Verification items for the finished model (mm, model axes). Coordinates: 2 decimals unless noted, no trailing zeros. Order: outer loops, then holes, each group sorted by start corner. A loop starts at its lowest first (then second) coordinate and runs counter-clockwise, first axis right, second up. Notation, with made-up numbers: (-23, 33) -> (9, 33) arc R28 ccw to (9, 54) -> close; hole circle Ø8 at (-31.75, 88.25). An arc over 180 degrees is marked (long way). Write each question's results on one line, items separated by ' | '. Start each with the question number.
(1) Go/stop test with a flat-tipped pin: pin 1 (6.5 mm diameter, centred on x = -41.5, z = 19.5, fed in from +Y). Record where the tip stops, or that it passes through.
(2) Cross-section at B-B on x = 0. Enter the section's corners in (y, z), and give its area (3 significant figures).
(3) Cross-section at C-C on z = 0. Enter the section's corners in (x, y), and give its area (3 significant figures).
(4) Cross-section at D-D on x = -41.5. Enter the section's corners in (y, z).
(5) Draft check along X on faces 1 (the cylindrical face through (-39.548, 24.65, 19.066)), 2 (the flat face through (-1, 25, -50)), 3 (the flat face through (-55, 25, 1)), 4 (the flat face through (55, 25, 1)). Enter one of: +X half, -X half, draft (parallel to the pull), parting line (faces both ways), or undercut.
(6) Thickness scan on probe 1 along Z at (x, y) = (-41.5, 24); probe 2 along X at (y, z) = (39, -19); probe 3 along X at (y, z) = (10, 0). Record the ranges inside material, lowest first. Write a range as [from, to].
(7) Cross-section at A-A on y = 25.5. Enter the section's corners in (x, z).
```python
from build123d import *

# Parameters (mm, degrees)
SKETCH1_W               = 110
SKETCH1_H               = 100
BOSS_EXTRUDE1_DEPTH     = 50
SKETCH2_R               = 35
CUT_EXTRUDE1_DEPTH      = 50
SKETCH3_R               = 2
CUT_EXTRUDE2_DEPTH      = 50
MIRROR3_COPY_1_SKETCH_R = 2
MIRROR3_COPY_1_DEPTH    = 50
MIRROR3_COPY_2_SKETCH_R = 2
MIRROR3_COPY_2_DEPTH    = 50


with BuildPart() as part:
    # Sketch1 → Boss-Extrude1 (new body)
    with BuildSketch(Plane(origin=(0, 0, 0), x_dir=(1, 0, 0), z_dir=(0, 1, 0))):
        Rectangle(SKETCH1_W, SKETCH1_H)
    extrude(amount=BOSS_EXTRUDE1_DEPTH)

    # Sketch2 → Cut-Extrude1 (cut)
    with BuildSketch(Plane(origin=(0, 0, 0), x_dir=(1, 0, 0), z_dir=(0, 1, 0))):
        with Locations(Location((0, 0, 0), (0, 0, 270))):
            Circle(SKETCH2_R)
    extrude(amount=CUT_EXTRUDE1_DEPTH, mode=Mode.SUBTRACT)

    # Sketch3 → Cut-Extrude2 (cut)
    with BuildSketch(Plane(origin=(0, 0, 0), x_dir=(1, 0, 0), z_dir=(0, 1, 0))):
        with Locations(Location((41.5, -19.5, 0), (0, 0, 270))):
            Circle(SKETCH3_R)
    cut_extrude2 = extrude(amount=CUT_EXTRUDE2_DEPTH, mode=Mode.SUBTRACT)

    # Mirror1: Cut-Extrude2 across plane
    add(cut_extrude2.mirror(Plane.XY), mode=Mode.SUBTRACT)

    # Mirror2: Cut-Extrude2 across plane
    add(cut_extrude2.mirror(Plane(origin=(0, 0, 0), x_dir=(0, 0, 1), z_dir=(1, 0, 0))), mode=Mode.SUBTRACT)

    # Mirror3 copy 1 sketch → Mirror3 copy 1 (cut)
    with BuildSketch(Plane(origin=(0, 0, 0), x_dir=(-1, 0, 0), z_dir=(0, 1, 0))):
        with Locations(Location((41.5, -19.5, 0), (0, 0, 270))):
            Circle(MIRROR3_COPY_1_SKETCH_R)
    extrude(amount=MIRROR3_COPY_1_DEPTH, mode=Mode.SUBTRACT)

    # Mirror3 copy 2 sketch → Mirror3 copy 2 (cut)
    with BuildSketch(Plane(origin=(0, 0, 0), x_dir=(1, 0, 0), z_dir=(0, 1, 0))):
        with Locations((41.5, 19.5)):
            Circle(MIRROR3_COPY_2_SKETCH_R)
    extrude(amount=MIRROR3_COPY_2_DEPTH, mode=Mode.SUBTRACT)


solid = part.part
```
Results are:
1) pin 1: stops at y = 50
2) outline: (0, -50) -> (50, -50) -> (50, -35) -> (0, -35) -> close; (0, 35) -> (50, 35) -> (50, 50) -> (0, 50) -> close | area: 1,500 mm2
3) outline: (-55, 0) -> (-35, 0) -> (-35, 50) -> (-55, 50) -> close; (35, 0) -> (55, 0) -> (55, 50) -> (35, 50) -> close | area: 2,000 mm2
4) outline: (0, -50) -> (50, -50) -> (50, -21.5) -> (0, -21.5) -> close; (0, -17.5) -> (50, -17.5) -> (50, 17.5) -> (0, 17.5) -> close; (0, 21.5) -> (50, 21.5) -> (50, 50) -> (0, 50) -> close
5) face 1: undercut | face 2: draft | face 3: -X half | face 4: +X half
6) probe 1: z = [-50, -21.5], [-17.5, 17.5], [21.5, 50] | probe 2: x = [-55, -43.44], [-39.56, -29.39], [29.39, 39.56], [43.44, 55] | probe 3: x = [-55, -35], [35, 55]
7) outline: (-55, -50) -> (55, -50) -> (55, 50) -> (-55, 50) -> close; hole circle Ø4 at (-41.5, -19.5); hole circle Ø4 at (-41.5, 19.5); hole circle Ø70 at (0, 0); hole circle Ø4 at (41.5, -19.5); hole circle Ø4 at (41.5, 19.5)
